Here's how the part is built. I have some questions about the finished solid (model axes, mm). Coordinates: 2 decimals unless noted, no trailing zeros. Write each loop counter-clockwise with the first axis right and the second up, starting at its lowest first coordinate (ties: lowest second). Pieces come first, ordered by that corner, then holes. Notation, with made-up numbers: M 79,57.25 L 137,57.25 A24 cw 137,67.25 Z; hole C 84.5,63.25 d8. An arc over 180 degrees is marked long. Use a Markdown table: item, result.
```python
from build123d import *

# Parameters (mm, degrees)
SKETCH1_W           = 20.06486665
SKETCH1_H           = 63.9
SKETCH1_R           = 3.35
BOSS_EXTRUDE1_DEPTH = 6.5
CHAMFER1_SIZE       = 1
SKETCH2_W           = 31.95
SKETCH2_H           = 3.25
CUT_EXTRUDE1_DEPTH  = 21.06486665


with BuildPart() as part:
    # Sketch1 → Boss-Extrude1 (new body)
    with BuildSketch(Plane(origin=(0, 0, 0), x_dir=(1, 0, 0), z_dir=(0, 1, 0))):
        with Locations((-10.582433325, -32.5)):
            Rectangle(SKETCH1_W, SKETCH1_H)
        with Locations((-10.582433325, -15.25)):
            Circle(SKETCH1_R, mode=Mode.SUBTRACT)
        with Locations((-10.582433325, -49.75)):
            Circle(SKETCH1_R, mode=Mode.SUBTRACT)
    extrude(amount=BOSS_EXTRUDE1_DEPTH)

    # Chamfer1
    chamfer1_edges = [part.edges().sort_by_distance(p)[0] for p in [
        (-13.932433325, 6.5, 15.25),
        (-13.932433325, 6.5, 49.75),
    ]]
    chamfer(chamfer1_edges, length=CHAMFER1_SIZE)

    # Sketch2 → Cut-Extrude1 (cut, through all)
    with BuildSketch(Plane(origin=(-0.55, 0, 0), x_dir=(0, 0, -1), z_dir=(1, 0, 0))):
        with Locations((-16.525, 1.625)):
            Rectangle(SKETCH2_W, SKETCH2_H)
    extrude(amount=-CUT_EXTRUDE1_DEPTH, mode=Mode.SUBTRACT)


solid = part.part
```
1. Suppose I cut it at C-C on z = 49.75. Write out the boundary of the cut face in (x, y), and give its area (3 significant figures).
Answers follow:
| item | result |
|---|---|
| outline | M -20.61,0 L -13.93,0 L -13.93,5.5 L -14.93,6.5 L -20.61,6.5 Z; M -7.23,0 L -0.55,0 L -0.55,6.5 L -6.23,6.5 L -7.23,5.5 Z |
| area | 85.9 mm2 |
2. Will these pins go through, and if not, where does the flat tip stop? pin 1 Ø3 at (x, z) = (-4.5, 32) entering from -Y; pin 2 Ø7.5 at (x, z) = (-10.58, 15.25) entering from +Y; pin 3 Ø1.5 at (x, y) = (-11, 1) entering from -Z.
Answers follow:
| item | result |
|---|---|
| pin 1 | stops at y = 0 |
| pin 2 | stops at y = 5.9 |
| pin 3 | stops at z = 32.5 |
3. I need wall thicknesses on probe 1 along X at (y, z) = (2.65, 49.75); probe 2 along Z at (x, y) = (-7.5, 3.75); probe 3 along Z at (x, y) = (-13.25, 4). Which ranges of each line are inside material? Lowest first, please.
Answers follow:
| item | result |
|---|---|
| probe 1 | x = -20.61 to -13.93, -7.23 to -0.55 |
| probe 2 | z = 0.55 to 13.94, 16.56 to 48.44, 51.06 to 64.45 |
| probe 3 | z = 0.55 to 13.22, 17.28 to 47.72, 51.78 to 64.45 |
4. Suppose I cut it at B-B on y = 1. Write out the boundary of the cut face in (x, z), and give its area (3 significant figures).
Answers follow:
| item | result |
|---|---|
| outline | M -20.61,32.5 L -0.55,32.5 L -0.55,64.45 L -20.61,64.45 Z; hole C -10.58,49.75 d6.7 |
| area | 606 mm2 |
5. Suppose I cut it at D-D on x = -2.25. Write out the boundary of the cut face in (y, z), and give its area (3 significant figures).
Answers follow:
| item | result |
|---|---|
| outline | M 0,32.5 L 3.25,32.5 L 3.25,0.55 L 6.5,0.55 L 6.5,64.45 L 0,64.45 Z |
| area | 312 mm2 |
6. Suppose I cut it at A-A on z = 15.25. Write out the boundary of the cut face in (x, y).
Answers follow:
| item | result |
|---|---|
| outline | M -20.61,3.25 L -13.93,3.25 L -13.93,5.5 L -14.93,6.5 L -20.61,6.5 Z; M -7.23,3.25 L -0.55,3.25 L -0.55,6.5 L -6.23,6.5 L -7.23,5.5 Z |
7. We'd pull the mould along Z, two halves only. Please class faces 1 (the face through (-11.31, 2.71, 53.02)), 2 (the face through (-10, 3.25, 20)), 3 (the face through (-10, 2, 32.5)), 4 (the face through (-13.052, 4.359, 12.986)): +Z half, -Z half, draft (parallel to the pull), parting line (faces both ways), or undercut.
Answers follow:
| item | result |
|---|---|
| face 1 | undercut |
| face 2 | draft |
| face 3 | -Z half |
| face 4 | undercut |
